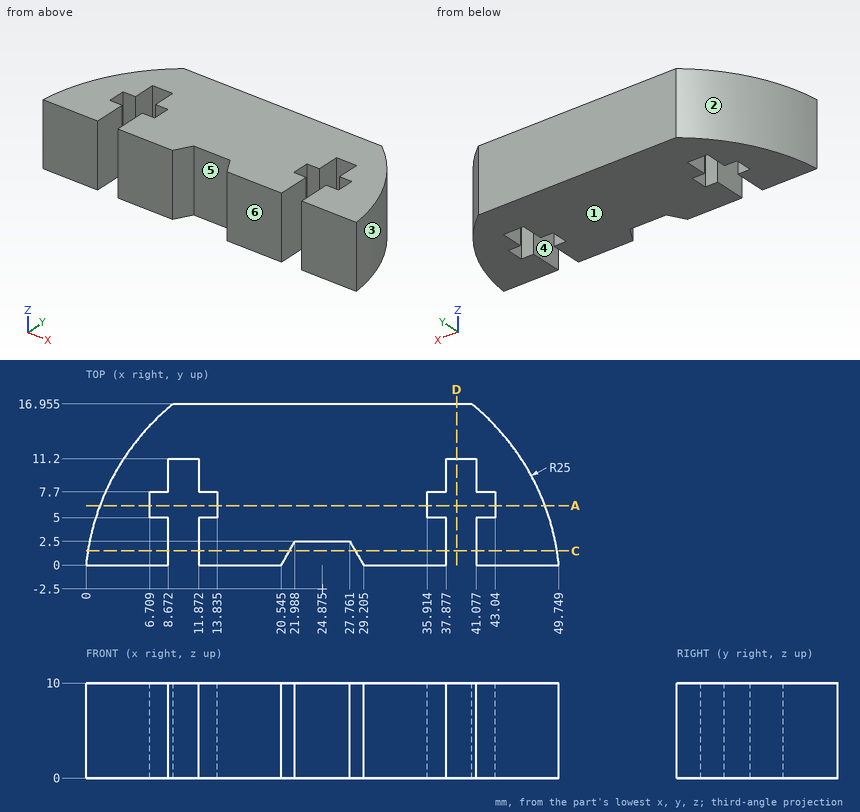
Source: three-view drawing plus pictorial views. Frame: mm from the lowest corner of the part. A direction names the side the tool comes from. Round coordinates to 2 decimals unless told otherwise and drop trailing zeros. Loops run counter-clockwise (first coordinate to the right, second up) from the corner with the lowest first, then second, coordinate; pieces in that order, holes last. Notation, with made-up numbers: M 82,69.5 L 91,69.5 A37 cw 91,108.5 Z; hole C 64.25,48.25 d10. An arc over 180 degrees is marked long. Put each result on its own line as item: value. Start each with the question number.
(1) Draft query along X for the marked faces 1, 2, 3 and 4. Return one class per face: +X half, -X half, draft (parallel to the pull), parting line (faces both ways), or undercut.
(2) Material intervals for line 1 along Y through (x, z) = (13, 4) (1 decimal); line 2 along X through (y, z) = (3.25, 7.5) (1 decimal); line 3 along X through (y, z) = (3.75, 9), sorted ascending. Write a range as [from, to].
(3) Section query C-C (y = 1.5). Return loops of the section in (x, z).
(4) Contact query for flat-ended pins moving along their axis: pin 1 Ø5.5 at (y, z) = (3, 3) entering from +X; pin 2 Ø5.5 at (y, z) = (3, 3.5) entering from -X; pin 3 Ø3 at (y, z) = (6, 6.5) entering from +X (1 decimal). Output: stop coordinate, or through.
(5) Section query A-A (y = 6.25). Return loops of the section in (x, z) (1 decimal).
(6) Set-up query: the marked faces 5 and 6. Return all of +Z, -Z, +X, -X, +Y, -Y with unobstructed straight access to the full face (end or side cutting, diameter ignored); none if empty.
(7) Section query D-D (x = 39). Return loops of the section in (y, z) (1 decimal).
Findings below:
1. face 1: draft
1. face 2: -X half
1. face 3: +X half
1. face 4: undercut
2. line 1: y = [0, 5], [7.7, 17]
2. line 2: x = [0.5, 8.7], [11.9, 37.9], [41.1, 49.2]
2. line 3: x = [0.67, 8.67], [11.87, 37.88], [41.08, 49.08]
3. outline: M 0.2,0 L 8.67,0 L 8.67,10 L 0.2,10 Z; M 11.87,0 L 21.41,0 L 21.41,10 L 11.87,10 Z; M 28.34,0 L 37.88,0 L 37.88,10 L 28.34,10 Z; M 41.08,0 L 49.55,0 L 49.55,10 L 41.08,10 Z
4. pin 1: stops at x = 49.72
4. pin 2: stops at x = 0.03
4. pin 3: stops at x = 48.9
5. outline: M 1.5,0 L 6.7,0 L 6.7,10 L 1.5,10 Z; M 13.8,0 L 35.9,0 L 35.9,10 L 13.8,10 Z; M 43,0 L 48.3,0 L 48.3,10 L 43,10 Z
6. face 5: +Z, -Z, -Y
6. face 6: +Z, -Z, +X, -X, -Y
7. outline: M 11.2,0 L 17,0 L 17,10 L 11.2,10 Z
